Could you check a few things on this model? Use its own coordinates, in mm. A direction names the side the tool comes from. Give positions to 0.01 mm unless a question says otherwise; leave off trailing zeros. Loops run counter-clockwise (first coordinate to the right, second up) from the corner with the lowest first, then second, coordinate; pieces in that order, holes last. Notation, with made-up numbers: M -16.75,-10 L 31.25,-10 A18 cw 31.25,0 Z; hole C 87,72 d10. An arc over 180 degrees is marked long. Return JSON: item names as keys, results as strings. Group by question number.
1. If we section it at B-B (z = 0): Write out the boundary of the cut face in (x, y), plus the area to 3 significant figures.
2. For pin 1 (8 mm diameter, centred on y = 591, z = 10.5, fed in from +X); pin 2 (10 mm diameter, centred on y = 347.5, z = 23.5, fed in from -X); pin 3 (2 mm diameter, centred on x = -63.5, y = 496.5, fed in from +Z); pin 4 (5 mm diameter, centred on y = 484.5, z = -38.5, fed in from +X), each with a flat end and sliding along its axis, tell me the tip position at first contact or that it passes through.
3. For faces 4 (the flat face through (-91, -29, 82.5)), 5 (the cylindrical face through (82.48, -28.59, 1.81)), 6 (the cylindrical face through (-7.94, -71.02, 99.79)), 7 (the flat face through (-1, -70.5, -152)), which set-ups out of +Z, -Z, +X, -X, +Y, -Y let a thin tool reach every point of the face, with its end or its side?
4. Please list where these lines run through material, in increasing order: line 1 (Y direction, x = -150, z = 70.25); line 2 (Z direction, x = -65, y = -169.5); line 3 (Y direction, x = 27.5, z = -92).
5. If we section it at A-A (y = -106): Write out the boundary of the cut face in (x, z).
6. If we section it at D-D (z = 117.5): Write out the boundary of the cut face in (x, y), plus the area to 3 significant figures.
7. If we mould it in two halves opening along X, with no side actions, what happens to faces 1 (the cylindrical face through (3.264, -238.836, -151.825)), 2 (the flat face through (-1, -70.5, 152)), 3 (the cylindrical face through (11.01, -190.18, -2.3))? For each: +X half, -X half, draft (parallel to the pull), parting line (faces both ways), or undercut.
8. If we section it at C-C (y = 340.5): Write out the boundary of the cut face in (x, z).
```python
from build123d import *

# Parameters (mm, degrees)
SKETCH1_R                = 61
BOSS_EXTRUDE1_DEPTH      = 815.982336818
BOSS_EXTRUDE2_DEPTH      = 58
CUT_EXTRUDE1_DEPTH       = 493
SKETCH3_3_R              = 18
CUT_EXTRUDE2_DEPTH       = 493
BOSS_EXTRUDE3_DEPTH      = 139.5
BOSS_EXTRUDE3_DEPTH_BACK = 139.5
SKETCH6_R                = 61
SKETCH7_R                = 106
BOSS_EXTRUDE5_DEPTH      = 25
CUT_EXTRUDE3_DEPTH       = 51
SKETCH9_R                = 72.5
BOSS_EXTRUDE6_DEPTH      = 141
SKETCH11_R               = 38.5
CUT_EXTRUDE6_DEPTH       = 450
SKETCH12_R               = 50.8
CUT_EXTRUDE7_DEPTH       = 630


with BuildPart() as part:
    # Sketch1 → Boss-Extrude1 (new body)
    with BuildSketch(Plane(origin=(0, 0, 0), x_dir=(1, 0, 0), z_dir=(0, 1, 0))):
        with Locations(Location((0, 0, 0), (0, 0, 270))):
            Circle(SKETCH1_R)
    extrude(amount=BOSS_EXTRUDE1_DEPTH)

    # Sketch2 → Boss-Extrude2 (add)
    with BuildSketch(Plane(origin=(0, 0, 0), x_dir=(-1, 0, 0), z_dir=(0, -1, 0))):
        with BuildLine():
            Line((0, 82.5), (179, 82.5))
            Line((179, 82.5), (179, 61.5))
            Line((179, 61.5), (54.990908339, 61.5))
            ThreePointArc((54.990908339, 61.5), (82.5, 0), (54.990908339, -61.5))
            Line((54.990908339, -61.5), (179, -61.5))
            Line((179, -61.5), (179, -82.5))
            Line((179, -82.5), (0, -82.5))
            ThreePointArc((0, -82.5), (-82.5, 0), (0, 82.5))
        make_face()
    extrude(amount=BOSS_EXTRUDE2_DEPTH)

    # Sketch3 → Cut-Extrude1 (cut)
    with BuildSketch(Plane(origin=(0, 0, -82.5), x_dir=(-1, 0, 0), z_dir=(0, 0, -1))):
        with BuildLine():
            Line((179, 0), (150, 0))
            ThreePointArc((150, 0), (170.506096654, -8.493903346), (179, -29))
            Line((179, -29), (179, 0))
        make_face()
        with BuildLine():
            ThreePointArc((179, -29), (170.506096654, -49.506096654), (150, -58))
            Line((150, -58), (179, -58))
            Line((179, -58), (179, -29))
        make_face()
    extrude(amount=-CUT_EXTRUDE1_DEPTH, mode=Mode.SUBTRACT)

    # Sketch3_3 → Cut-Extrude2 (cut)
    with BuildSketch(Plane(origin=(0, 0, -82.5), x_dir=(-1, 0, 0), z_dir=(0, 0, -1))):
        with Locations((150, -29)):
            Circle(SKETCH3_3_R)
    extrude(amount=-CUT_EXTRUDE2_DEPTH, mode=Mode.SUBTRACT)



with BuildPart() as body_2:
    # Sketch6 → Boss-Extrude3 (new, two sides: drawn at the far end of the back side and taken through both)
    with BuildSketch(Plane.XY.offset(-BOSS_EXTRUDE3_DEPTH_BACK)):
        with Locations((0, -131.5)):
            Circle(SKETCH6_R)
    extrude(amount=BOSS_EXTRUDE3_DEPTH + BOSS_EXTRUDE3_DEPTH_BACK)

    # Sketch7 → Boss-Extrude5 (add)
    with BuildSketch(Plane(origin=(0, 0, -139.5), x_dir=(-1, 0, 0), z_dir=(0, 0, -1))):
        with Locations((0, -132.886327958)):
            Circle(SKETCH7_R)
    boss_extrude5 = extrude(amount=BOSS_EXTRUDE5_DEPTH)

    # Sketch8 → Cut-Extrude3 (cut)
    with BuildSketch(Plane.XY.offset(-139.5)):
        Polygon((0, -70.5), (144.590777868, -70.5), (144.590777868, 11.025223161), (-136.314365489, 11.025223161), (-136.314365489, -70.5), align=None)
    cut_extrude3 = extrude(amount=-CUT_EXTRUDE3_DEPTH, mode=Mode.SUBTRACT)

    # Mirror1: Boss-Extrude5, Cut-Extrude3 across plane
    add(boss_extrude5.mirror(Plane.XY))
    add(cut_extrude3.mirror(Plane.XY), mode=Mode.SUBTRACT)


with BuildPart() as part_1:
    add(part.part)

    add(body_2.part)  # Boss-Extrude6 merges body 2
    # Sketch9 → Boss-Extrude6 (add)
    with BuildSketch(Plane.XZ.offset(58)):
        with Locations(Location((0, 0, 0), (0, 0, 270))):
            Circle(SKETCH9_R)
    extrude(amount=BOSS_EXTRUDE6_DEPTH)

    # Sketch11 → Cut-Extrude6 (cut)
    with BuildSketch(Plane(origin=(0, 0, -164.5), x_dir=(-1, 0, 0), z_dir=(0, 0, -1))):
        with Locations((0, -141.739564151)):
            Circle(SKETCH11_R)
    extrude(amount=-CUT_EXTRUDE6_DEPTH, mode=Mode.SUBTRACT)

    # Sketch12 → Cut-Extrude7 (cut)
    with BuildSketch(Plane(origin=(0, 0, -164.5), x_dir=(-1, 0, 0), z_dir=(0, 0, -1))):
        with Locations((0, -140.586472034)):
            Circle(SKETCH12_R)
    extrude(amount=-CUT_EXTRUDE7_DEPTH, mode=Mode.SUBTRACT)


solid = part_1.part
```
Answer:
{
 "1": {"outline": "M -82.5,-58 L -72.5,-58 L -72.5,-199 L 72.5,-199 L 72.5,-58 L 82.5,-58 L 82.5,0 L 61,0 L 61,815.98 L -61,815.98 L -61,0 L -82.5,0 Z; hole C 0,-140.59 d101.6", "area": "121,000 mm²"},
 "2": {"pin 1": "stops at x = 60.65", "pin 2": "stops at x = -58.13", "pin 3": "passes through", "pin 4": "stops at x = 49.24"},
 "3": {"face 4": "+Z, +X, -X, +Y", "face 5": "+X, +Y", "face 6": "none", "face 7": "-Z, +X, -X, +Y"},
 "4": {"line 1": "y = -58 to -47, -11 to 0", "line 2": "z = -164.5 to -139.5, -32.11 to 32.11, 139.5 to 164.5", "line 3": "y = -185.95 to -183.3, -97.87 to -77.05"},
 "5": {"outline": "M -102.53,-164.5 L -37.21,-164.5 L -37.21,164.5 L -102.53,164.5 L -102.53,139.5 L -55.41,139.5 L -55.41,46.75 A72.5 ccw -55.41,-46.75 L -55.41,-139.5 L -102.53,-139.5 Z; M 37.21,-164.5 L 102.53,-164.5 L 102.53,-139.5 L 55.41,-139.5 L 55.41,-46.75 A72.5 ccw 55.41,46.75 L 55.41,139.5 L 102.53,139.5 L 102.53,164.5 L 37.21,164.5 Z"},
 "6": {"outline": "C 0,-131.5 d122; hole C 0,-140.59 d101.6", "area": "3,580 mm²"},
 "7": {"face 1": "parting line", "face 2": "draft", "face 3": "undercut"},
 "8": {"outline": "C 0,0 d122"}
}
